Part model, mm, in its own coordinate system. A direction names the side the tool comes from. Give positions to 0.01 mm unless a question says otherwise; leave off trailing zeros. Order: outer loops, then holes, each group sorted by start corner. A loop starts at its lowest first (then second) coordinate and runs counter-clockwise, first axis right, second up. Notation, with made-up numbers: M 62.25,-8.75 L 88.25,-8.75 A26 ccw 88.25,24.25 Z; hole C 84,86.5 d7. An arc over 180 degrees is marked long. Write each question's results on one line, items separated by ' | '. Start each with the question number.
Autodesk Inventor part; units mm, degrees
ref_plane "YZ Plane" through (0, 0, 0) normal (1, 0, 0) x (0, 1, 0)
ref_plane "XZ Plane" through (0, 0, 0) normal (0, 1, 0) x (-1, 0, 0)
ref_plane "XY Plane" through (0, 0, 0) normal (0, 0, 1) x (1, 0, 0)
sketch "Sketch1" plane through (0, 0, 0) normal (0, 0, 1) x (1, 0, 0)
  line L0 (0, 0) -> (552.45, 0)
  line L1 (552.45, 0) -> (552.45, 127)
  line L2 (552.45, 127) -> (0, 127)
  line L3 (0, 127) -> (0, 0)
  dimension "d0" = 552.45
  dimension "d1" = 127
extrude "Extrusion1" add sketch "Sketch1" against normal blind 6.35
sketch "Sketch2" plane through (0, 0, 0) normal (0, 0, 1) x (1, 0, 0)
  line L0 (552.45, 0) -> (552.45, 127)
  line L1 (552.45, 127) -> (0, 127)
  line L2 (0, 127) -> (0, 0)
  line L3 (315.976, 25.4) -> (315.976, 101.6)
  arc A0 (315.976, 101.6) -> (293.624, 101.6) centre (304.8, 101.6) ccw
  line L4 (293.624, 101.6) -> (293.624, 25.4)
  arc A1 (293.624, 25.4) -> (315.976, 25.4) centre (304.8, 25.4) ccw
  point P0 (276.225, 127)
  dimension "d4" = 76.2
  dimension "d6" = 11.176
  dimension "d7" = 247.65
  dimension "d8" = 25.4
extrude "Extrusion2" cut sketch "Sketch2" against normal up to next
properties part number "GE_13030" material "Polyethylene, High Density"
(1) Tool access for faces 1 (the cylindrical face through (304.554, 14.227, -3.131)), 2 (the flat face through (272, 64, 0)): list every direction of +Z, -Z, +X, -X, +Y, -Y with a clear straight run to the whole face (end or side of a thin tool).
(2) Saw through at A-A on x = 304.8. Give the cut face in (y, z).
(3) Pull direction Y, two halves, no side cores. Call faces 3 (the flat face through (272, 64, -6.35)), 4 (the cylindrical face through (305.046, 112.773, -3.131)): +Y half, -Y half, draft (parallel to the pull), parting line (faces both ways), or undercut.
(4) Saw through at B-B on y = 83.5. Give the cut face in (x, z).
(5) Saw through at C-C on z = -2. Give the cut face in (x, y), plus the area to 3 significant figures.
(6) Probe L1, parallel to X at y = 37, z = -4.5; L2, parallel to X at y = 20, z = -4.75. List the from-to ranges inside material, lowest first.
Taken from the geometry:
1) face 1: +Z, -Z | face 2: +Z, +X, -X, +Y, -Y
2) outline: M 0,-6.35 L 14.22,-6.35 L 14.22,0 L 0,0 Z; M 112.78,-6.35 L 127,-6.35 L 127,0 L 112.78,0 Z
3) face 3: draft | face 4: undercut
4) outline: M 0,-6.35 L 293.62,-6.35 L 293.62,0 L 0,0 Z; M 315.98,-6.35 L 552.45,-6.35 L 552.45,0 L 315.98,0 Z
5) outline: M 0,0 L 552.45,0 L 552.45,127 L 0,127 Z; hole M 293.62,25.4 A11.18 ccw 315.98,25.4 L 315.98,101.6 A11.18 ccw 293.62,101.6 Z | area: 68,100 mm²
6) L1: x = 0 to 293.62, 315.98 to 552.45 | L2: x = 0 to 295.02, 314.58 to 552.45
